```python
from build123d import *

# Parameters (mm, degrees)
BOSS_EXTRUDE1_DEPTH = 12
SKETCH2_R           = 19.5
SKETCH2_R_2         = 3.5
BOSS_EXTRUDE2_DEPTH = 4
SKETCH3_R           = 3.5
CUT_EXTRUDE1_DEPTH  = 12


with BuildPart() as part:
    # Sketch1 → Boss-Extrude1 (new body)
    with BuildSketch(Plane.XY):
        Polygon((-23, 25), (23, 25), (31, 0), (23, -25), (-23, -25), (-31, 0), align=None)
    extrude(amount=BOSS_EXTRUDE1_DEPTH)

    # Sketch2 → Boss-Extrude2 (add)
    with BuildSketch(Plane.XY.offset(12)):
        Circle(SKETCH2_R)
        with Locations((23.75, 0)):
            Circle(SKETCH2_R_2)
        with Locations((-23.75, 0)):
            Circle(SKETCH2_R_2)
    extrude(amount=BOSS_EXTRUDE2_DEPTH)

    # Sketch3 → Cut-Extrude1 (cut)
    with BuildSketch(Plane.XY.offset(12)):
        with Locations((18.25, 18.25)):
            Circle(SKETCH3_R)
        with Locations((18.25, -18.25)):
            Circle(SKETCH3_R)
        with Locations((-18.25, -18.25)):
            Circle(SKETCH3_R)
        with Locations((-18.25, 18.25)):
            Circle(SKETCH3_R)
    extrude(amount=-CUT_EXTRUDE1_DEPTH, mode=Mode.SUBTRACT)


solid = part.part
```
Design review of the part built by this model. Coordinates are the model's own, in mm. A direction names the side the tool comes from. Round coordinates to 2 decimals unless told otherwise and drop trailing zeros. Write each loop counter-clockwise with the first axis right and the second up, starting at its lowest first coordinate (ties: lowest second). Pieces come first, ordered by that corner, then holes.
Item 1: We need section B-B on x = -21. Write out the cut boundary in (y, z), and give its area (3 significant figures).
Item 2: We need section A-A on y = -7.5. Write out the cut boundary in (x, z), and give its area (3 significant figures).
Item 3: Clearance check with flat-ended pins moving along their axes: pin 1 Ø4 at (x, y) = (2, -14) entering from -Z; pin 2 Ø1 at (y, z) = (1.5, 13.5) entering from +X; pin 3 Ø4 at (x, y) = (18.25, -18.25) entering from +Z; pin 4 Ø1 at (y, z) = (17, 7.5) entering from +X. State where each tip first meets the part, or that it passes through.
Item 4: The part is to be moulded in two halves that separate along X. For faces 3 (the cylindrical face through (27.09, 1.05, 13.97)), 4 (the flat face through (24, 0, 16)), 5 (the flat face through (-27.056, 12.325, 5.916)), 6 (the flat face through (27.056, -12.325, 5.916)), say which applies: +X half, -X half, draft (parallel to the pull), parting line (faces both ways), or undercut.
Item 5: For faces 1 (the flat face through (-26.944, -12.675, 5.916)), 2 (the flat face through (-20, 0, 12)), list the 3-axis set-ups (+Z, -Z, +X, -X, +Y, -Y) from which the entire face can be reached by the end or side of a thin tool; tool diameter is ignored.
Item 6: For probe 1 along Y at (x, z) = (18.25, 9.25); probe 2 along X at (y, z) = (-19.5, 11.5); probe 3 along X at (y, z) = (21, 4.75), list the stretches that pass through material, from the lowest coordinate up.
Item 7: We need section C-C on z = 9.75. Write out the cut boundary in (x, y), and give its area (3 significant figures).
Item 8: We need section D-D on y = -18.25. Write out the cut boundary in (x, z).
Returned:
1. outline: (-25, 0) - (-20.42, 0) - (-20.42, 12) - (-25, 12) - close; (-16.08, 0) - (16.08, 0) - (16.08, 12) - (2.17, 12) - (2.17, 16) - (-2.17, 16) - (-2.17, 12) - (-16.08, 12) - close; (20.42, 0) - (25, 0) - (25, 12) - (20.42, 12) - close
1. area: 513 mm2
2. outline: (-28.6, 0) - (28.6, 0) - (28.6, 12) - (18, 12) - (18, 16) - (-18, 16) - (-18, 12) - (-28.6, 12) - close
2. area: 830 mm2
3. pin 1: stops at z = 0
3. pin 2: stops at x = 27.1
3. pin 3: passes through
3. pin 4: stops at x = 25.72
4. face 3: undercut
4. face 4: draft
4. face 5: -X half
4. face 6: +X half
5. face 1: +Z, -Z, -X, -Y
5. face 2: +Z
6. probe 1: y = -25 to -21.75, -14.75 to 14.75, 21.75 to 25
6. probe 2: x = -24.76 to -21.52, -14.98 to 14.98, 21.52 to 24.76
6. probe 3: x = -24.28 to -20.42, -16.08 to 16.08, 20.42 to 24.28
7. outline: (-31, 0) - (-23, -25) - (23, -25) - (31, 0) - (23, 25) - (-23, 25) - close; hole circle Ø7 at (-18.25, -18.25); hole circle Ø7 at (-18.25, 18.25); hole circle Ø7 at (18.25, -18.25); hole circle Ø7 at (18.25, 18.25)
7. area: 2,550 mm2
8. outline: (-25.16, 0) - (-21.75, 0) - (-21.75, 12) - (-25.16, 12) - close; (-14.75, 0) - (14.75, 0) - (14.75, 12) - (6.87, 12) - (6.87, 16) - (-6.87, 16) - (-6.87, 12) - (-14.75, 12) - close; (21.75, 0) - (25.16, 0) - (25.16, 12) - (21.75, 12) - close
